```python
from build123d import *

# Parameters (mm, degrees)
F0_R     = 2
F1_DEPTH = 3
F2_W     = 19.86
F2_H     = 24
F2_H_2   = 3
F3_DEPTH = 3
F4_W     = 20
F4_H     = 2.75
F5_DEPTH = 2.75
F6_W     = 20
F6_H     = 1.9
F7_DEPTH = 1.9
F8_DEPTH = 2


with BuildPart() as f1:
    # F0 (on Top) → F1 (new body)
    with BuildSketch(Plane.XY):
        Polygon((-44.965, -13.73), (44.965, -13.73), (44.965, 13.73), (-20.755, 13.73), (-20.755, 4.94), (-25.105, 4.94), (-25.105, 13.73), (-44.965, 13.73), align=None)
        with Locations((39.595, -5.23)):
            Circle(F0_R, mode=Mode.SUBTRACT)
        with Locations((-39.365, 5.1)):
            Circle(F0_R, mode=Mode.SUBTRACT)
    extrude(amount=F1_DEPTH)

    # F2 (on face) → F3 (join)
    with BuildSketch(Plane(origin=(0, 13.73, 0), x_dir=(-1, 0, 0), z_dir=(0, 1, 0))):
        Polygon((11.269, 0), (20.755, 0), (20.755, 3), (20.755, 27), (-44.965, 27), (-44.965, 3), (-44.965, 0), (-8.731, 0), align=None)
        with Locations((35.035, 15)):
            Rectangle(F2_W, F2_H)
        with Locations((35.035, 1.5)):
            Rectangle(F2_W, F2_H_2)
    extrude(amount=F3_DEPTH)

    # F4 (on face) → F5 (join)
    with BuildSketch(Plane(origin=(0, 16.73, 0), x_dir=(-1, 0, 0), z_dir=(0, 1, 0))):
        with Locations((1.269, 21.625)):
            Rectangle(F4_W, F4_H)
    extrude(amount=F5_DEPTH)

    # F6 (on face) → F7 (join)
    with BuildSketch(Plane(origin=(0, 19.48, 0), x_dir=(-1, 0, 0), z_dir=(0, 1, 0))):
        Polygon((11.269, 20.25), (-8.731, 20.25), (-8.731, 18.5663476586), (-4.159652628, 18.27), (0.319, 18.27), (0.519, 19.52), (4.269, 19.52), (4.269, 18.27), (11.269, 18.27), align=None)
        Polygon((-8.731, 23), (-8.731, 20.25), (11.269, 20.25), (11.269, 21.625), (11.269, 23), align=None)
        with Locations((1.269, 23.95)):
            Rectangle(F6_W, F6_H)
    extrude(amount=F7_DEPTH)

    # F2 (on face) → F8 (join)
    with BuildSketch(Plane(origin=(0, 13.73, 0), x_dir=(-1, 0, 0), z_dir=(0, 1, 0))):
        with Locations((35.035, 15)):
            Rectangle(F2_W, F2_H)
        Polygon((11.269, 0), (20.755, 0), (20.755, 3), (20.755, 27), (-44.965, 27), (-44.965, 3), (-44.965, 0), (-8.731, 0), align=None)
    extrude(amount=-F8_DEPTH)


solid = f1.part
```
The listing builds one solid part. Answer for the finished solid, in the listing's coordinates (mm). A direction names the side the tool comes from. Give positions to 0.01 mm unless a question says otherwise; leave off trailing zeros. Order: outer loops, then holes, each group sorted by start corner. A loop starts at its lowest first (then second) coordinate and runs counter-clockwise, first axis right, second up. Notation, with made-up numbers: (6, -2) - (49, -2) arc R21 cw to (49, 20) - close; hole circle Ø3 at (22.5, 30). An arc over 180 degrees is marked (long way). Answer in a Markdown table with one row per item. Add a question column.
Q1. Given P1, Ø2, axis at x = 21, y = 0, coming from the +Z side; P2, Ø1.6, axis at x = -6, z = 19, coming from the -Y side; P3, Ø4, axis at x = -3.5, z = 14, coming from the +Y side, each flat-ended and moving along its own axis, determine where each tip first touches the part or whether it passes through.
Q2. For a pull along X with two mould halves and no side action, classify faces 5 (the flat face through (-20.755, 13, 13)), 6 (the flat face through (6.48, 20.42, 18.42)), 7 (the cylindrical face through (41.503, -4.629, 1.479)), 8 (the flat face through (-35, 11.73, 15)) as released by +X, released by -X, zero draft, split by the parting line, or undercut.
Q3. The part is cut by section A-A (y = 8). Determine the outline of the cut face in (x, z) (3 decimals).
Q4. The part is cut by section B-B (z = 11.75). Determine the outline of the cut face in (x, y) (3 decimals), then the cut area to 3 significant figures.
Q5. The part is cut by section D-D (x = 36). Determine the outline of the cut face in (y, z).
Q6. Which of the six approach directions +Z, -Z, +X, -X, +Y, -Y give full straight-line access (tool end or side, diameter ignored) to faces 1 (the flat face through (-2, 20, 19.52)), 2 (the flat face through (-1, 18, 23)), 3 (the flat face through (-1, -1, 3)), 4 (the flat face through (-23, 4.94, 1))?
Q7. The part is cut by section C-C (x = -7.5). Determine the outline of the cut face in (y, z), then the cut area to 3 significant figures.
Q8. Find the intervals of material crossed by line 1 along X through (y, z) = (15.5, 26.25) (3 decimals); line 2 along Y through (x, z) = (19, 12.75); line 3 along Z through (x, y) = (10.5, -7.5), in increasing order. Write a range as [from, to].
Determined:
| question | item | result |
|---|---|---|
| 1 | P1 | stops at z = 3 |
| 1 | P2 | stops at y = 11.73 |
| 1 | P3 | stops at y = 16.73 |
| 2 | face 5 | undercut |
| 2 | face 6 | released by +X |
| 2 | face 7 | undercut |
| 2 | face 8 | zero draft |
| 3 | outline | (-44.965, 0) - (-25.105, 0) - (-25.105, 3) - (-44.965, 3) - close; (-20.755, 0) - (44.965, 0) - (44.965, 3) - (-20.755, 3) - close |
| 4 | outline | (-44.965, 11.73) - (-25.105, 11.73) - (-25.105, 16.73) - (-44.965, 16.73) - close; (-20.755, 11.73) - (44.965, 11.73) - (44.965, 16.73) - (-20.755, 16.73) - close |
| 4 | area | 428 mm² |
| 5 | outline | (-13.73, 0) - (16.73, 0) - (16.73, 27) - (11.73, 27) - (11.73, 3) - (-13.73, 3) - close |
| 6 | face 1 | -Z, +Y |
| 6 | face 2 | +Z, +X, -X |
| 6 | face 3 | +Z, +X, -X, -Y |
| 6 | face 4 | +Z, -Z, +Y |
| 7 | outline | (-13.73, 0) - (16.73, 0) - (16.73, 20.25) - (19.48, 20.25) - (19.48, 18.27) - (21.38, 18.27) - (21.38, 24.9) - (19.48, 24.9) - (19.48, 23) - (16.73, 23) - (16.73, 27) - (11.73, 27) - (11.73, 3) - (-13.73, 3) - close |
| 7 | area | 232 mm² |
| 8 | line 1 | x = [-44.965, -25.105], [-20.755, 44.965] |
| 8 | line 2 | y = [11.73, 16.73] |
| 8 | line 3 | z = [0, 3] |
